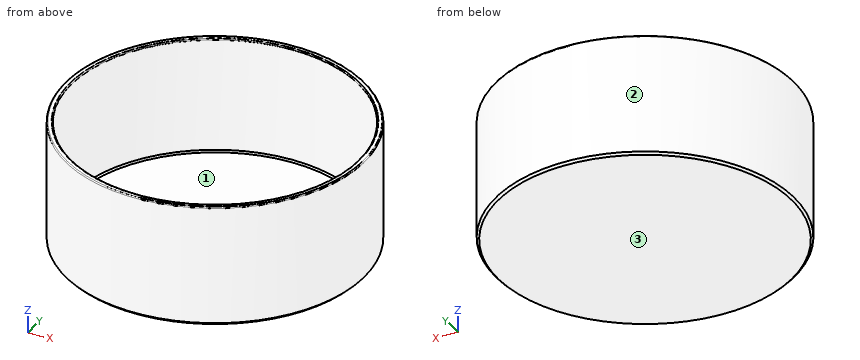
```python
from build123d import *

# Parameters (mm, degrees)
F0_R     = 67.5
F1_DEPTH = 55
F2_T     = -2.5
F3_R     = 0.5
F4_SIZE  = 1
F5_SIZE  = 0.75


with BuildPart() as f1:
    # F0 (on Top) → F1 (new body)
    with BuildSketch(Plane.XY):
        Circle(F0_R)
    extrude(amount=F1_DEPTH)

    # F2
    f2_openings = [f1.faces().sort_by_distance(p)[0] for p in [
        (0, 0, 55),
    ]]
    offset(amount=F2_T, openings=f2_openings)

    # F3
    f3_edges = [f1.edges().sort_by_distance(p)[0] for p in [
        (-67.5, 0, 55),
        (-65, 0, 55),
    ]]
    fillet(f3_edges, radius=F3_R)

    # F4
    f4_edges = [f1.edges().sort_by_distance(p)[0] for p in [
        (-67.5, 0, 0),
    ]]
    chamfer(f4_edges, length=F4_SIZE)

    # F5
    f5_edges = [f1.edges().sort_by_distance(p)[0] for p in [
        (-65, 0, 2.5),
    ]]
    chamfer(f5_edges, length=F5_SIZE)


solid = f1.part
```
Verification items for the finished model (mm, model axes). Face numbers are marked on the shaded views. Give positions to 0.01 mm unless a question says otherwise; leave off trailing zeros. Order: outer loops, then holes, each group sorted by start corner. A loop starts at its lowest first (then second) coordinate and runs counter-clockwise, first axis right, second up. Notation, with made-up numbers: M 71,24.5 L 93,24.5 A24 cw 93,44.5 Z; hole C 83.25,-5 d3. An arc over 180 degrees is marked long. Return JSON: item names as keys, results as strings. Group by question number.
1) Section check A-A on x = 0. Record the cut outline in (y, z).
2) Scan lines: line 1 (Y direction, x = 0, z = 28); line 2 (Z direction, x = 49, y = -13); line 3 (Y direction, x = 54.5, z = 34). Record each from-to range of solid material in increasing order.
3) Section check C-C on z = 18. Record the cut outline in (x, y), and give its area (3 significant figures).
4) Go/stop test with flat-tipped pins: pin 1 Ø3 at (y, z) = (-4.5, 10.5) entering from +X; pin 2 Ø4 at (y, z) = (-9, 15) entering from -X; pin 3 Ø1 at (y, z) = (48, 17.5) entering from +X. Record where each tip stops, or that it passes through.
5) Mould release check, pull along Y, two halves, no side actions. Record for the marked faces 1, 2 and 3: pulls with the +Y half, pulls with the -Y half, needs draft (parallel to the pull), parting line crosses it, or undercut.
Answer block:
{
 "1": {"outline": "M -67.5,1 L -66.5,0 L 66.5,0 L 67.5,1 L 67.5,54.5 A0.5 ccw 67,55 L 65.5,55 A0.5 ccw 65,54.5 L 65,3.25 L 64.25,2.5 L -64.25,2.5 L -65,3.25 L -65,54.5 A0.5 ccw -65.5,55 L -67,55 A0.5 ccw -67.5,54.5 Z"},
 "2": {"line 1": "y = -67.5 to -65, 65 to 67.5", "line 2": "z = 0 to 2.5", "line 3": "y = -39.82 to -35.42, 35.42 to 39.82"},
 "3": {"outline": "C 0,0 d135; hole C 0,0 d130", "area": "1,040 mm^2"},
 "4": {"pin 1": "stops at x = 67.43", "pin 2": "stops at x = -67.14", "pin 3": "stops at x = 47.96"},
 "5": {"face 1": "undercut", "face 2": "parting line crosses it", "face 3": "needs draft"}
}
